Part model, mm, in its own coordinate system. Coordinates: 2 decimals unless noted, no trailing zeros. Order: outer loops, then holes, each group sorted by start corner. A loop starts at its lowest first (then second) coordinate and runs counter-clockwise, first axis right, second up. Notation, with made-up numbers: (-15.75, 8) - (40.25, 8) arc R8 cw to (40.25, 22) - close; hole circle Ø4 at (-4, 72.25). An arc over 180 degrees is marked (long way). Use a Markdown table: item, result. Add a question column.
1) Saw through at B-B on x = -8. List the corners of the cut face in (y, z) (3 decimals), then the cut area to 3 significant figures.
2) Saw through at C-C on y = 0.35. List the corners of the cut face in (x, z) (3 decimals).
3) Drop a flat-ended pin along its axis: P1, Ø1, axis at x = -11.5, z = -6.5, coming from the -Y side. Give the stop position or say it passes through.
4) Wall check: L1, parallel to X at y = 0.4, z = 0 (3 decimals); L2, parallel to X at y = 1.25, z = -7.5; L3, parallel to Z at x = -1.5, y = 1.15. Give the ranges that are in metal, low to high. Write a range as [from, to].
5) Two-plate mould, pull along Z, no slides. Class faces 1 (the face through (6.755, 0.811, -0.276)), 2 (the face through (16.855, 0.789, -2.213)), 3 (the face through (0, 1.6, 0)): +Z half, -Z half, draft (parallel to the pull), parting line (faces both ways), or undercut.
6) Saw through at D-D on x = 0. List the corners of the cut face in (y, z) (3 decimals), then the cut area to 3 significant figures.
7) Saw through at A-A on z = 0. List the corners of the cut face in (x, y) (3 decimals).
```python
from build123d import *

# Parameters (mm, degrees)
SKETCH_1_R          = 17
EXTRUDE_1_DEPTH     = 1.6
SKETCH_2_R          = 1.275
CUT_EXTRUDE_1_DEPTH = 25.09481272


with BuildPart() as part:
    # 草图1 → 凸台-拉伸1 (new body)
    with BuildSketch(Plane(origin=(0, 0, 0), x_dir=(1, 0, 0), z_dir=(0, 1, 0))):
        with Locations(Location((0, 0, 0), (0, 0, 270))):
            Circle(SKETCH_1_R)
    extrude(amount=EXTRUDE_1_DEPTH)

    # 草图2 → 切除-拉伸1 (cut, through all)
    with BuildSketch(Plane(origin=(0, 1.6, 0), x_dir=(1, 0, 0), z_dir=(0, 1, 0))):
        with Locations(Location((8, 0, 0), (0, 0, 270))):
            Circle(SKETCH_2_R)
        with Locations(Location((0, -8, 0), (0, 0, 270))):
            Circle(SKETCH_2_R)
        with Locations(Location((-8, 0, 0), (0, 0, 270))):
            Circle(SKETCH_2_R)
        with Locations(Location((0, 8, 0), (0, 0, 270))):
            Circle(SKETCH_2_R)
    extrude(amount=-CUT_EXTRUDE_1_DEPTH, mode=Mode.SUBTRACT)


solid = part.part
```
Results are:
| question | item | result |
|---|---|---|
| 1 | outline | (0, -15) - (1.6, -15) - (1.6, -1.275) - (0, -1.275) - close; (0, 1.275) - (1.6, 1.275) - (1.6, 15) - (0, 15) - close |
| 1 | area | 43.9 mm2 |
| 2 | outline | circle Ø34 at (0, 0); hole circle Ø2.55 at (-8, 0); hole circle Ø2.55 at (0, -8); hole circle Ø2.55 at (0, 8); hole circle Ø2.55 at (8, 0) |
| 3 | P1 | y = 0 |
| 4 | L1 | [-17, -9.275], [-6.725, 6.725], [9.275, 17] |
| 4 | L2 | [-15.26, -1.17], [1.17, 15.26] |
| 4 | L3 | [-16.93, 16.93] |
| 5 | face 1 | undercut |
| 5 | face 2 | parting line |
| 5 | face 3 | draft |
| 6 | outline | (0, -17) - (1.6, -17) - (1.6, -9.275) - (0, -9.275) - close; (0, -6.725) - (1.6, -6.725) - (1.6, 6.725) - (0, 6.725) - close; (0, 9.275) - (1.6, 9.275) - (1.6, 17) - (0, 17) - close |
| 6 | area | 46.2 mm2 |
| 7 | outline | (-17, 0) - (-9.275, 0) - (-9.275, 1.6) - (-17, 1.6) - close; (-6.725, 0) - (6.725, 0) - (6.725, 1.6) - (-6.725, 1.6) - close; (9.275, 0) - (17, 0) - (17, 1.6) - (9.275, 1.6) - close |
